Geometry check sheet. Reference: drawing and pictorial views, mm from the part's lowest x, y, z. Coordinates: 2 decimals unless noted, no trailing zeros. Write each loop counter-clockwise with the first axis right and the second up, starting at its lowest first coordinate (ties: lowest second). Pieces come first, ordered by that corner, then holes. Notation, with made-up numbers: (75.25, 6) - (115.25, 6) arc R31 ccw to (115.25, 34) - close; hole circle Ø5 at (-5.5, 80.5). An arc over 180 degrees is marked (long way). Use one line per item in the form item = value. Start each with the question number.
(1) Material ranges on line 1 (X direction, y = 4, z = 1.75) (1 decimal); line 2 (Y direction, x = 68.5, z = 1.85), recorded low to high. Write a range as [from, to].
(2) Sectioned sample at B-B (y = 5). Record the cut outline in (x, z) (1 decimal).
(3) Sectioned sample at A-A (z = 1.7). Count the separate pieces of the cut face and the enclosed holes in it.
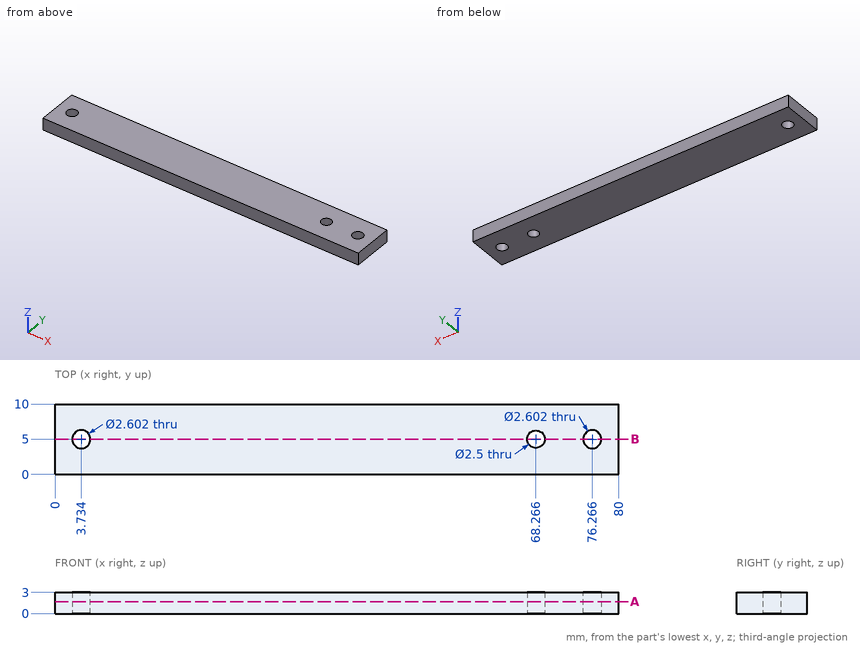
Answers below:
q1.line_1 = [0, 2.9], [4.6, 67.5], [69, 75.4], [77.1, 80]
q1.line_2 = [0, 3.77], [6.23, 10]
q2.outline = (0, 0) - (2.4, 0) - (2.4, 3) - (0, 3) - close; (5, 0) - (67, 0) - (67, 3) - (5, 3) - close; (69.5, 0) - (75, 0) - (75, 3) - (69.5, 3) - close; (77.6, 0) - (80, 0) - (80, 3) - (77.6, 3) - close
q3.separate_pieces = 1
q3.enclosed_holes = 3
